Design review of the part built by this model. Coordinates are the model's own, in mm. A direction names the side the tool comes from. Round coordinates to 2 decimals unless told otherwise and drop trailing zeros. Order: outer loops, then holes, each group sorted by start corner. A loop starts at its lowest first (then second) coordinate and runs counter-clockwise, first axis right, second up. Notation, with made-up numbers: M 36.5,18.5 L 42.5,18.5 A22 cw 42.5,47.5 Z; hole C 43,-5 d3. An arc over 180 degrees is marked long. Write item = value, one per line. Start each with the question number.
```python
from build123d import *

# Parameters (mm, degrees)
SKETCH1_W           = 22.83
SKETCH1_H           = 12.22
BOSS_EXTRUDE1_DEPTH = 17.35
BOSS_EXTRUDE2_DEPTH = 2.47
SKETCH3_W           = 22.63
SKETCH3_H           = 12.22
BOSS_EXTRUDE3_DEPTH = 4.1
BOSS_EXTRUDE4_DEPTH = 4.1
SKETCH5_R           = 2.375
BOSS_EXTRUDE5_DEPTH = 3.8


with BuildPart() as part:
    # Sketch1 → Boss-Extrude1 (new body)
    with BuildSketch(Plane(origin=(0, 0, 0), x_dir=(1, 0, 0), z_dir=(0, 1, 0))):
        with Locations((11.415, 6.11)):
            Rectangle(SKETCH1_W, SKETCH1_H)
    extrude(amount=BOSS_EXTRUDE1_DEPTH)

    # Sketch2 → Boss-Extrude2 (add)
    with BuildSketch(Plane(origin=(0, 17.35, 0), x_dir=(1, 0, 0), z_dir=(0, 1, 0))):
        with BuildLine():
            Line((-4.715, 0), (27.545, 0))
            Line((27.545, 0), (27.545, 5.61))
            Line((27.545, 5.61), (26.709213562, 5.61))
            ThreePointArc((26.709213562, 5.61), (23.795, 6.11), (26.709213562, 6.61))
            Line((26.709213562, 6.61), (27.545, 6.61))
            Line((27.545, 6.61), (27.545, 12.22))
            Line((27.545, 12.22), (-4.715, 12.22))
            Line((-4.715, 12.22), (-4.715, 6.61))
            Line((-4.715, 6.61), (-3.879213562, 6.61))
            ThreePointArc((-3.879213562, 6.61), (-0.965, 6.11), (-3.879213562, 5.61))
            Line((-3.879213562, 5.61), (-4.715, 5.61))
            Line((-4.715, 5.61), (-4.715, 0))
        make_face()
    extrude(amount=BOSS_EXTRUDE2_DEPTH)

    # Sketch3 → Boss-Extrude3 (add)
    with BuildSketch(Plane(origin=(0, 19.82, 0), x_dir=(1, 0, 0), z_dir=(0, 1, 0))):
        with Locations((11.415, 6.11)):
            Rectangle(SKETCH3_W, SKETCH3_H)
    extrude(amount=BOSS_EXTRUDE3_DEPTH)

    # Sketch4 → Boss-Extrude4 (add)
    with BuildSketch(Plane(origin=(0, 23.92, 0), x_dir=(1, 0, 0), z_dir=(0, 1, 0))):
        with BuildLine():
            Line((12.32, 3.36), (11.666152491, 3.36))
            ThreePointArc((11.666152491, 3.36), (0.1, 6.11), (11.666152491, 8.86))
            Line((11.666152491, 8.86), (12.32, 8.86))
            ThreePointArc((12.32, 8.86), (15.07, 6.11), (12.32, 3.36))
        make_face()
    extrude(amount=BOSS_EXTRUDE4_DEPTH)

    # Sketch5 → Boss-Extrude5 (add)
    with BuildSketch(Plane(origin=(0, 28.02, 0), x_dir=(1, 0, 0), z_dir=(0, 1, 0))):
        with Locations(Location((6.21, 6.11, 0), (0, 0, 90))):
            Circle(SKETCH5_R)
    extrude(amount=BOSS_EXTRUDE5_DEPTH)


solid = part.part
```
(1) Consider section A-A, the plane z = -5. Write out the cut boundary in (x, y) (3 decimals).
(2) Consider section D-D, the plane z = -9.25. Write out the cut boundary in (x, y) (3 decimals), then the cut area to 3 significant figures.
(3) For faces 1 (the face through (6.106, 29.893, -3.737)), 2 (the face through (27, 19, -5.61)), 3 (the face through (18, 23.92, -6)), 4 (the face through (22.83, 9, -6)), 5 (the face through (22.73, 22, -6)), list the 3-axis set-ups (+Z, -Z, +X, -X, +Y, -Y) from which the entire face can be reached by the end or side of a thin tool; tool diameter is ignored.
(4) Consider section B-B, the plane x = 0.5. Write out the cut boundary in (y, z), then the cut area to 3 significant figures.
(5) For line 1 along Y through (x, z) = (11, -1); line 2 along Y through (x, z) = (7.5, -0.5); line 3 along X through (y, z) = (7, -10.75), list the stretches that pass through material, from the lowest coordinate up. Write a range as [from, to].
(6) Draft analysis for pull direction X (two halves, no side actions). For faces 6 (the face through (-0.966, 18.568, -6.169)), 7 (the face through (25, 17.35, -8)), 8 (the face through (23.796, 18.568, -6.051)), 9 (the face through (0.1, 22, -6)), state which applies: pulls with the +X half, pulls with the -X half, needs draft (parallel to the pull), parting line crosses it, or undercut.
(7) Consider section C-C, the plane y = 25. Write out the cut boundary in (x, z).
(8) Insertion check: pin 1 (1 mm diameter, centred on x = 24, y = 8, fed in from -Z); pin 2 (10 mm diameter, centred on x = 5.5, y = 28, fed in from +Z); pin 3 (5 mm diameter, centred on x = 1.5, z = -10.5, fed in from +Y); pin 4 (0.5 mm diameter, centred on x = 12, y = 26.5, fed in from +Z). Each pin has a flat end and moves straight along its axis. Give the tip position at first contact, or say it passes through.
Completed:
q1.outline = M -4.715,17.35 L -3.474,17.35 L -3.474,19.82 L -4.715,19.82 Z; M -1.456,17.35 L 0,17.35 L 0,0 L 22.83,0 L 22.83,17.35 L 24.286,17.35 L 24.286,19.82 L 22.73,19.82 L 22.73,23.92 L 14.836,23.92 L 14.836,28.02 L 8.31,28.02 L 8.31,31.82 L 4.11,31.82 L 4.11,28.02 L 0.202,28.02 L 0.202,23.92 L 0.1,23.92 L 0.1,19.82 L -1.456,19.82 Z; M 26.304,17.35 L 27.545,17.35 L 27.545,19.82 L 26.304,19.82 Z
q2.outline = M -4.715,17.35 L 0,17.35 L 0,0 L 22.83,0 L 22.83,17.35 L 27.545,17.35 L 27.545,19.82 L 22.73,19.82 L 22.73,23.92 L 11.451,23.92 L 11.451,28.02 L 0.969,28.02 L 0.969,23.92 L 0.1,23.92 L 0.1,19.82 L -4.715,19.82 Z
q2.area = 612 mm2
q3.face_1 = +Y
q3.face_2 = +X, +Y, -Y
q3.face_3 = +X, +Y
q3.face_4 = +Z, -Z, +X, -Y
q3.face_5 = +Z, -Z, +X, +Y
q4.outline = M 0,-12.22 L 23.92,-12.22 L 23.92,-8.28 L 28.02,-8.28 L 28.02,-3.94 L 23.92,-3.94 L 23.92,0 L 0,0 Z
q4.area = 310 mm2
q5.line_1 = [0, 23.92]
q5.line_2 = [0, 28.02]
q5.line_3 = [0, 22.83]
q6.face_6 = undercut
q6.face_7 = needs draft
q6.face_8 = undercut
q6.face_9 = pulls with the -X half
q7.outline = M 11.67,-8.86 L 12.32,-8.86 A2.75 ccw 12.32,-3.36 L 11.67,-3.36 A6.11 ccw long Z
q8.pin_1 = through
q8.pin_2 = 0
q8.pin_3 = 28.02
q8.pin_4 = -3.36
